```python
from build123d import *

# Parameters (mm, degrees)
F1_DEPTH = 60
F2_R     = 3.375
F3_DEPTH = 15
F4_R     = 2


with BuildPart() as f1:
    # F0 (on Right) → F1 (new body)
    with BuildSketch(Plane.YZ):
        with BuildLine():
            Line((0, 0), (0, -35.67515))
            Line((0, -35.67515), (20, -35.67515))
            Line((20, -35.67515), (20, 0))
            Line((20, 0), (12.194061, 8.370845))
            ThreePointArc((12.194061, 8.370845), (10, 9.32485), (7.805939, 8.370845))
            Line((7.805939, 8.370845), (0, 0))
        make_face()
    extrude(amount=F1_DEPTH)

    # F2 (on face) → F3 (cut)
    with BuildSketch(Plane(origin=(0, 0, -35.67515), x_dir=(1, 0, 0), z_dir=(0, 0, -1))):
        with Locations((8.993604, -10)):
            Circle(F2_R)
        with Locations((51.006395, -10)):
            Circle(F2_R)
    extrude(amount=-F3_DEPTH, mode=Mode.SUBTRACT)

    # F4
    f4_edges = [f1.edges().sort_by_distance(p)[0] for p in [
        (30, 20, -35.67515),
        (30, 0, -35.67515),
    ]]
    fillet(f4_edges, radius=F4_R)


solid = f1.part
```
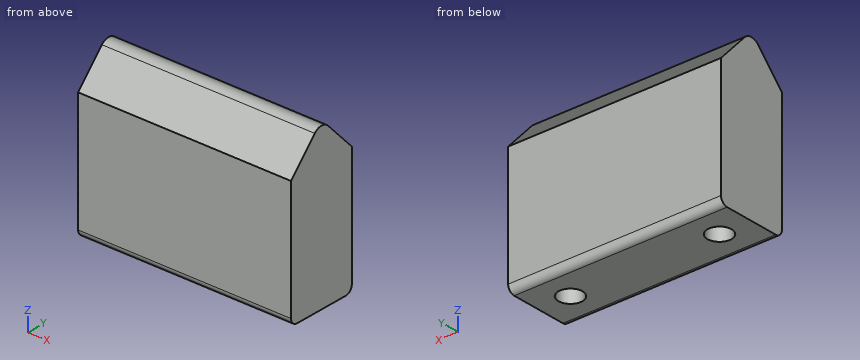
CAD build for the part. Positions are in the model's coordinates, mm. Coordinates: 2 decimals unless noted, no trailing zeros. Order: outer loops, then holes, each group sorted by start corner. A loop starts at its lowest first (then second) coordinate and runs counter-clockwise, first axis right, second up. Notation, with made-up numbers: (-26.5, -37.75) - (-9.5, -37.75) arc R19 cw to (-9.5, -15.75) - close; hole circle Ø6 at (-11, 6.25). An arc over 180 degrees is marked (long way). Use a Markdown table: item, result. Add a question column.
(1) Drill centre lines: line 1 along X through (y, z) = (10, -29.25); line 2 along Z through (x, y) = (27.5, 12); line 3 along Y through (x, z) = (13, 5). Where is each one in solid material? Low to high. Write a range as [from, to].
(2) Saw through at D-D (x = 53). Give the cut face in (y, z), then the cut area to 3 significant figures.
(3) Saw through at A-A (y = 10). Give the cut face in (x, z), then the cut area to 3 significant figures.
(4) Saw through at C-C (z = 5.5). Give the cut face in (x, y), then the cut area to 3 significant figures.
(5) Saw through at B-B (x = 40). Give the cut face in (y, z).
(6) Flat gauge pins, fed straight in: pin 1 (3 mm diameter, centred on x = 24, z = 4.5, fed in from -Y); pin 2 (3.5 mm diameter, centred on x = 51.5, y = 11, fed in from -Z); pin 3 (8 mm diameter, centred on x = 41, y = 17.5, fed in from +Z). Where does each tip first touch, or does it go through?
Solved:
| question | item | result |
|---|---|---|
| 1 | line 1 | x = [0, 5.62], [12.37, 47.63], [54.38, 60] |
| 1 | line 2 | z = [-35.68, 8.56] |
| 1 | line 3 | y = [4.66, 15.34] |
| 2 | outline | (0, -33.68) arc R2 ccw to (2, -35.68) - (7.28, -35.68) - (7.28, -20.68) - (12.72, -20.68) - (12.72, -35.68) - (18, -35.68) arc R2 ccw to (20, -33.68) - (20, 0) - (12.19, 8.37) arc R3 ccw to (7.81, 8.37) - (0, 0) - close |
| 2 | area | 735 mm² |
| 3 | outline | (0, -35.68) - (5.62, -35.68) - (5.62, -20.68) - (12.37, -20.68) - (12.37, -35.68) - (47.63, -35.68) - (47.63, -20.68) - (54.38, -20.68) - (54.38, -35.68) - (60, -35.68) - (60, 9.32) - (0, 9.32) - close |
| 3 | area | 2,500 mm² |
| 4 | outline | (0, 5.13) - (60, 5.13) - (60, 14.87) - (0, 14.87) - close |
| 4 | area | 585 mm² |
| 5 | outline | (0, -33.68) arc R2 ccw to (2, -35.68) - (18, -35.68) arc R2 ccw to (20, -33.68) - (20, 0) - (12.19, 8.37) arc R3 ccw to (7.81, 8.37) - (0, 0) - close |
| 6 | pin 1 | stops at y = 2.8 |
| 6 | pin 2 | stops at z = -20.68 |
| 6 | pin 3 | stops at z = 6.97 |
